Solid Edge part; units mm, degrees
sketch "Sketch1" plane through (0, 0, 0) normal (0, 0, 1) x (1, 0, 0)
  line L0 (-6, -1.3) -> (6, -1.3)
  line L1 (6, -1.3) -> (6, 1.3)
  line L2 (6, 1.3) -> (-6, 1.3)
  line L3 (-6, 1.3) -> (-6, -1.3)
  dimension "D1" = 6
extrude "Protrusion1" add sketch "Sketch1" along normal mid plane 2.6
sketch "Sketch2" plane through (6, 0, 0) normal (1, 0, 0) x (0, 1, 0)
  line L0 (-0.3, -0.3) -> (0.3, -0.3)
  line L1 (0.3, -0.3) -> (0.3, 0.3)
  line L2 (0.3, 0.3) -> (-0.3, 0.3)
  line L3 (-0.3, 0.3) -> (-0.3, -0.3)
  dimension "D1" = 0.3
  dimension "D2" = 0.3
extrude "Extrusionsausschnitt_1" cut sketch "Sketch2" against normal blind 5.5
chamfer "Fase_1" distance 0.5 angle 45 4 edges at (6, 0, 0.3) (6, 0.3, 0) (6, -0.3, 0) (6, 0, -0.3)
sketch "Sketch3" plane through (-6, 0, 0) normal (-1, 0, 0) x (0, -1, 0)
  circle A0 centre (0, 0) radius 0.75
extrude "Extrusionsausschnitt_2" cut sketch "Sketch3" against normal blind 5.5
sketch "Sketch4" plane through (0, 0, 1.3) normal (0, 0, 1) x (1, 0, 0)
  line L0 (0.2, -1.3) -> (-3.4, -1.3)
  line L1 (-3.4, -1.3) -> (-3.4, -0.7966)
  line L2 (-3.4, -0.7966) -> (0.2, -0.7966)
  line L3 (0.2, 0.8) -> (0.2, -0.7966)
  line L4 (-3.4, 0.8) -> (0.2, 0.8)
  line L5 (-3.4, 1.3) -> (-3.4, 0.8)
  line L6 (0.2, 1.3) -> (-3.4, 1.3)
  line L7 (2.4, 1.3) -> (0.2, 1.3)
  line L8 (2.4, -1.3) -> (2.4, 1.3)
  line L9 (0.2, -1.3) -> (2.4, -1.3)
  dimension "D1" = 2.4
  dimension "D2" = 3.4
  dimension "D3" = 3.4
  dimension "D4" = 0.2
extrude "Extrusionsausschnitt_3" cut sketch "Sketch4" against normal blind 0.1
sketch "Sketch5" plane through (-0.5, 0, 1.2) normal (0, 0, 1) x (1, 0, 0)
  line L0 (0.8, 0.8) -> (2.8, 0.8)
  line L1 (2.8, 0.8) -> (2.8, -0.8)
  line L2 (2.8, -0.8) -> (0.8, -0.8)
  line L3 (0.8, -0.8) -> (0.8, 0.8)
  dimension "D1" = 0.8
extrude "Extrusionsausschnitt_4" cut sketch "Sketch5" against normal blind 0.1
sketch "Sketch6" plane through (6, 0, 0) normal (1, 0, 0) x (0, 0, -1)
  line L0 (-0.3, -0.3) -> (0.3, -0.3)
  line L1 (0.3, -0.3) -> (0.3, 0.3)
  line L2 (0.3, 0.3) -> (-0.3, 0.3)
  line L3 (-0.3, 0.3) -> (-0.3, -0.3)
extrude "Extrusionsausprägung_2" add sketch "Sketch6" against normal blind 5.5 and the other way blind 5.5
chamfer "Fase_2" distance 0.25 angle 45 2 edges at (11.5, 0, 0.3) (11.5, 0, -0.3)
fillet "Verrundung_1" radius 0.1 10 edges at (11.5, 0, 0.05) (11.5, 0, -0.05) (11.25, 0, 0.3) (11.25, 0, -0.3) (11.375, -0.3, -0.175) (11.375, -0.3, 0.175) (11.5, -0.3, 0) (11.375, 0.3, 0.175) (11.5, 0.3, 0) (11.375, 0.3, -0.175)
chamfer "Fase_3" distance 0.25 angle 45 1 edges at (-6, 0.75, 0)
Check sheet for the modelled part. Datum: model origin and axes. Units: mm. A direction names the side the tool comes from. Round coordinates to 2 decimals unless told otherwise and drop trailing zeros. One line per question, with ' | ' between items. Start each with the question number.
1. Depth check by flat-ended pin: pin 1 (0.5 mm diameter, centred on x = 7, z = 0, fed in from -Y); pin 2 (0.8 mm diameter, centred on y = 0, z = 0.5, fed in from -X); pin 3 (0.5 mm diameter, centred on x = 9, z = 0, fed in from +Y). Enter the tip coordinate at first touch or a pass-through.
2. Release check for a two-part mould opening along Z. For faces 4 (the face through (4, 0, 1.3)), 5 (the face through (0, 0, -1.3)), 6 (the face through (-6, 1, -1)), 7 (the face through (-0.5, 0, 0)) record: +Z half, -Z half, draft (parallel to the pull), parting line (faces both ways), or undercut.
3. Set-up check for faces 1 (the face through (1, 0, 1.1)), 2 (the face through (0, -1.3, 0)), 3 (the face through (-3.16, 0.75, 0.03)): record each of +Z, -Z, +X, -X, +Y, -Y from which the full face is reachable in a straight line by a thin tool's end or side.
4. Scan lines: line 1 along Z through (x, y) = (-2.8, 0); line 2 along X through (y, z) = (-1, 0.15); line 3 along Y through (x, z) = (10.75, 0.1). Record each from-to range of solid material in increasing order. Write a range as from..to.
Taken from the geometry:
1) pin 1: stops at y = -0.3 | pin 2: stops at x = -5.9 | pin 3: stops at y = 0.3
2) face 4: +Z half | face 5: -Z half | face 6: draft | face 7: undercut
3) face 1: +Z | face 2: +Z, -Z, +X, -X, -Y | face 3: -X
4) line 1: z = -1.3..-0.75, 0.75..1.3 | line 2: x = -6..6 | line 3: y = -0.3..0.3
